Autodesk Inventor part; units mm, degrees
ref_plane "YZ Plane" through (0, 0, 0) normal (1, 0, 0) x (0, 1, 0)
ref_plane "XZ Plane" through (0, 0, 0) normal (0, 1, 0) x (-1, 0, 0)
ref_plane "XY Plane" through (0, 0, 0) normal (0, 0, 1) x (1, 0, 0)
sketch "Sketch24" plane through (0, 0, 0) normal (0, 1, 0) x (-1, 0, 0)
  line L0 (-17.5, 14.75) -> (17.5, 14.75)
  line L1 (17.5, 14.75) -> (17.5, -14.75)
  line L2 (17.5, -14.75) -> (-17.5, -14.75)
  line L3 (-17.5, -14.75) -> (-17.5, 14.75)
  line L4 (-17.5, 14.75) -> (17.5, -14.75) construction
  line L5 (17.5, 14.75) -> (-17.5, -14.75) construction
  line L6 (-9.3, 8.2) -> (9.3, 8.2)
  line L7 (12.3, 5.2) -> (12.3, -5.2)
  line L8 (9.3, -8.2) -> (-9.3, -8.2)
  line L9 (-12.3, -5.2) -> (-12.3, 5.2)
  line L10 (-12.3, 8.2) -> (12.3, -8.2) construction
  line L11 (12.3, 8.2) -> (-12.3, -8.2) construction
  arc A0 (12.3, 5.2) -> (9.3, 8.2) centre (9.3, 5.2) ccw
  arc A1 (9.3, -8.2) -> (12.3, -5.2) centre (9.3, -5.2) ccw
  arc A2 (-12.3, -5.2) -> (-9.3, -8.2) centre (-9.3, -5.2) ccw
  arc A3 (-9.3, 8.2) -> (-12.3, 5.2) centre (-9.3, 5.2) ccw
  circle A4 centre (0, 0) radius 12.25
  dimension "d54" = 35
  dimension "d55" = 29.5
  dimension "d56" = 16.4
  dimension "d57" = 24.6
  dimension "d58" = 3
  dimension "d59" = 24.5
extrude "Extrusion20" add sketch "Sketch24" along normal blind 19.5 contours L0 L1 L2 L3 | L6 A4 L8 A2 L9 A3 | A4 L6 | L6 A4 L8 | L6 A0 L7 A1 L8 A4 | L8 A4
extrude "Extrusion21" cut sketch "Sketch24" along normal blind 3.8 contours L6 A4 L8 A2 L9 A3 | L6 A4 L8 | L6 A0 L7 A1 L8 A4
sketch "Sketch25" plane through (0, 19.5, 0) normal (0, 1, 0) x (1, 0, 0)
  line L0 (9, 5) -> (-9, -5) construction
  point P0 (0, 0)
  point P1 (9, -5)
  point P2 (-9, 5)
  point P3 (0, 0)
  dimension "d71" = 10
  dimension "d72" = 18
hole "Hole1" at (9, 19.5, -5) at (-9, 19.5, 5) direction (0, -1, 0) diameter 2.6 end through all counterbore diameter 5.5 counterbore depth 2.9
sketch "Sketch26" plane through (0, 3.8, 0) normal (0, -1, 0) x (1, 0, 0)
  circle A0 centre (0, 0) radius 6
  dimension "d73" = 12
extrude "Extrusion22" cut sketch "Sketch26" against normal through all
sketch "Sketch27" plane through (-17.5, 0, 14.75) normal (0, 0, 1) x (1, 0, 0)
  line L0 (0, 0) -> (35, 0)
  line L1 (0, 19.5) -> (35, 19.5)
  point P0 (17.5, 0)
  point P1 (29.5, 11)
  point P2 (5.5, 11)
  point P3 (17.5, 0)
  point P4 (17.5, 0)
  point P5 (0, 11)
  dimension "d83" = 12
  dimension "d84" = 12
  dimension "d145" = 8.5
hole "Hole2" at (12, 11, 14.75) at (-12, 11, 14.75) direction (0, 0, -1) diameter 2.459 depth 9 tip angle 118
sketch "Sketch28" plane through (17.5, 0, -14.75) normal (0, 0, -1) x (-1, 0, 0)
  circle A0 centre (29.5, 11) radius 1.2295
  circle A1 centre (5.5, 11) radius 1.2295
  point P0 (17.5, 0)
hole "Hole3" at (-12, 11, -14.75) at (12, 11, -14.75) direction (0, 0, 1) diameter 2.459 depth 9 tip angle 118
sketch "Sketch29" plane through (0, 3.8, 0) normal (0, -1, 0) x (1, 0, 0)
  line L0 (-9, -5.5) -> (-9, 1.5) construction
  line L1 (-7.5, -5.5) -> (-7.5, 1.5)
  line L2 (-10.5, 1.5) -> (-10.5, -5.5)
  arc A0 (-10.5, -5.5) -> (-7.5, -5.5) centre (-9, -5.5) ccw
  arc A1 (-7.5, 1.5) -> (-10.5, 1.5) centre (-9, 1.5) ccw
  line L3 (9, -1.5) -> (9, 5.5) construction
  line L4 (10.5, -1.5) -> (10.5, 5.5)
  line L5 (7.5, 5.5) -> (7.5, -1.5)
  arc A2 (7.5, -1.5) -> (10.5, -1.5) centre (9, -1.5) ccw
  arc A3 (10.5, 5.5) -> (7.5, 5.5) centre (9, 5.5) ccw
  point P0 (0, 0)
  point P1 (-9, -2)
  point P2 (9, 2)
  point P3 (-9, 3)
  point P4 (-9, -7)
  dimension "d94" = 3
  dimension "d95" = 10
  dimension "d96" = 1.5
  dimension "d97" = 9
  dimension "d98" = 9
  dimension "d99" = 1.5
extrude "Extrusion23" cut sketch "Sketch29" against normal blind 2.5
sketch "Sketch30" plane through (0, 6.3, 0) normal (0, -1, 0) x (1, 0, 0)
  arc A0 (-10.5, -5.5) -> (-7.5, -5.5) centre (-9, -5.5) ccw
  arc A1 (10.5, 5.5) -> (7.5, 5.5) centre (9, 5.5) ccw
  point P0 (0, 0)
hole "Hole4" at (-9, 6.3, -5.5) at (9, 6.3, 5.5) direction (0, 1, 0) diameter 2.5 end through all
sketch "Sketch31" plane through (0, 6.3, 0) normal (0, -1, 0) x (1, 0, 0)
  arc A0 (-7.5, 1.5) -> (-10.5, 1.5) centre (-9, 1.5) ccw
  arc A1 (7.5, -1.5) -> (10.5, -1.5) centre (9, -1.5) ccw
  point P0 (0, 0)
  point P1 (-9, 0)
  point P2 (9, 0)
  point P3 (9, 0)
  point P4 (-9, 3)
hole "Hole5" at (-9, 6.3, 0) at (9, 6.3, 0) direction (0, 1, 0) diameter 2.013 end through all
sketch "Sketch32" plane through (0, 19.5, 0) normal (0, 1, 0) x (1, 0, 0)
  circle A0 centre (-9, 0) radius 1.0065
  circle A1 centre (9, 0) radius 1.0065
  point P0 (0, 0)
  point P1 (-9.5915, -2.3144)
  point P2 (-8.4085, -2.3144)
  point P3 (9.5915, 2.3144)
  point P4 (8.4085, 2.3144)
hole "Hole6" at (-9, 19.5, 0) at (9, 19.5, 0) direction (0, -1, 0) diameter 3.3 depth 7 tip angle 118
sketch "Sketch33" plane through (0, 19.5, 0) normal (0, 1, 0) x (1, 0, 0)
  point P0 (0, 0)
  point P1 (0, -10)
  point P2 (0, 10)
  dimension "d131" = 10
  dimension "d132" = 10
hole "Hole7" at (0, 19.5, 10) at (0, 19.5, -10) direction (0, -1, 0) diameter 3.1 end through all counterbore diameter 6.5 counterbore depth 3.4
sketch "Sketch35" plane through (0, 0, 0) normal (0, -1, 0) x (1, 0, 0)
  line L0 (50, -2) -> (0, -2)
  line L1 (0, -2) -> (0, 2)
  line L2 (0, 2) -> (50, 2)
  line L3 (50, 2) -> (50, -2)
  point P0 (0, 0)
  point P1 (0, 0)
  dimension "d138" = 4
  dimension "d139" = 50
extrude "Extrusion24" cut sketch "Sketch35" against normal blind 3.8
pattern_circular "Circular Pattern1" count 3 over 360 about axis through (0, 3.8, 0) along (0, 1, 0) of "Extrusion24"
properties material "Copper"
Verification items for the finished model (mm, model axes). A direction names the side the tool comes from. Give positions to 0.01 mm unless a question says otherwise; leave off trailing zeros. Write each loop counter-clockwise with the first axis right and the second up, starting at its lowest first coordinate (ties: lowest second). Pieces come first, ordered by that corner, then holes. Notation, with made-up numbers: M 24,72 L 46,72 A23 ccw 46,91 Z; hole C 49.5,69.5 d6. An arc over 180 degrees is marked long. Use CSV: the item, a comma, the result in double quotes.
1) Material ranges on line 1 along Z through (x, y) = (-9, 7.5); line 2 along Z through (x, y) = (0, 8); line 3 along X through (y, z) = (15.5, 0), recorded low to high.
Final values:
line 1,"-14.75 to -6.75, -4.25 to -1.01, 1.01 to 3.7, 6.3 to 14.75"
line 2,"-14.75 to -11.55, -8.45 to -6, 6 to 8.45, 11.55 to 14.75"
line 3,"-17.5 to -10.65, -7.35 to -6, 6 to 7.35, 10.65 to 17.5"
2) Cross-section at D-D (y = 14). State how many separate pieces and enclosed holes the cut face has, plus the area to 3 significant figures.
Final values:
separate pieces,"1"
enclosed holes,"9"
area,"867 mm²"
3) Cross-section at B-B (y = 5.75). Enter the section's corners in (x, z).
Final values:
outline,"M -17.5,-14.75 L 17.5,-14.75 L 17.5,14.75 L -17.5,14.75 Z; hole M -10.5,-5.5 A1.5 ccw -7.5,-5.5 L -7.5,1.5 A1.5 ccw -10.5,1.5 Z; hole C -9,5 d2.6; hole C 0,0 d12; hole C 0,-10 d3.1; hole C 0,10 d3.1; hole M 7.5,-1.5 A1.5 ccw 10.5,-1.5 L 10.5,5.5 A1.5 ccw 7.5,5.5 Z; hole C 9,-5 d2.6"
4) Cross-section at C-C (z = -10). Enter the section's corners in (x, y), plus the area to 3 significant figures.
Final values:
outline,"M -17.5,0 L -8.08,0 L -8.08,3.8 L -3.46,3.8 L -3.46,0 L -1.55,0 L -1.55,16.1 L -3.25,16.1 L -3.25,19.5 L -17.5,19.5 Z; M 1.55,0 L 17.5,0 L 17.5,19.5 L 3.25,19.5 L 3.25,16.1 L 1.55,16.1 Z; hole C -12,11 d2.46; hole C 12,11 d2.46"
area,"583 mm²"
5) Go/stop test with flat-tipped pins: pin 1 Ø3 at (x, z) = (5, 5) entering from -Y; pin 2 Ø1.2 at (x, z) = (-9, 0) entering from -Y; pin 3 Ø0.7 at (x, y) = (-7.5, 1.5) entering from -Z; pin 4 Ø1.5 at (x, z) = (-8.5, 0) entering from -Y. Record where each tip stops, or that it passes through.
Final values:
pin 1,"y = 3.8"
pin 2,"through"
pin 3,"z = -9.6"
pin 4,"y = 6.3"
6) Access from +Z, -Z, +X, -X, +Y, -Y to the whole of each face (thin tool, end or side, straight path). Record for faces 5 (the face through (-10.29, 10.11, 4.83)), 6 (the face through (12.3, 2, -4)), 7 (the face through (-9.83, 18.03, 7.62)), 8 (the face through (-12.369, 9.827, 10.187)), 9 (the face through (15, 2, -2)).
Final values:
face 5,"+Y, -Y"
face 6,"-Y"
face 7,"+Y"
face 8,"+Z"
face 9,"+X, -Y"
7) Cross-section at A-A (y = 2). Enter the section's corners in (x, z).
Final values:
outline,"M -17.5,-14.75 L -10.83,-14.75 L -7.04,-8.2 L -9.3,-8.2 A3 cw -12.3,-5.2 L -12.3,5.2 A3 cw -9.3,8.2 L -7.04,8.2 L -10.83,14.75 L -17.5,14.75 Z; M -6.21,-14.75 L 17.5,-14.75 L 17.5,-2 L 12.3,-2 L 12.3,-5.2 A3 cw 9.3,-8.2 L -2.42,-8.2 Z; M -6.21,14.75 L -2.42,8.2 L 9.3,8.2 A3 cw 12.3,5.2 L 12.3,2 L 17.5,2 L 17.5,14.75 Z; hole C 0,-10 d3.1; hole C 0,10 d3.1"
8) Release check for a two-part mould opening along Z. For faces 1 (the face through (8, 0, -10)), 2 (the face through (0, 10, -14.75)), 3 (the face through (-10.5, 5, -2)), 4 (the face through (12.009, 11.213, 5.14)) record: released by +Z, released by -Z, zero draft, split by the parting line, or undercut.
Final values:
face 1,"zero draft"
face 2,"released by -Z"
face 3,"undercut"
face 4,"released by +Z"
